Source: CAD feature listing. Evaluate the final solid. Frame: model axes, mm. A direction names the side the tool comes from. Coordinates: 2 decimals unless noted, no trailing zeros. Loops run counter-clockwise (first coordinate to the right, second up) from the corner with the lowest first, then second, coordinate; pieces in that order, holes last. Notation, with made-up numbers: M 6.25,27.5 L 60.25,27.5 A5 cw 60.25,32.5 Z; hole C -2.5,18.25 d11. An arc over 180 degrees is marked long. One line per question, with ' | ' between items. Start each with the question number.
1. Access query for faces 4 (the cylindrical face through (158.805, 91.82, 1.463)), 5 (the cylindrical face through (86.417, 17.759, 0.986)). Directions: +Z, -Z, +X, -X, +Y, -Y. A direction counts if a zero-diameter tool reaches every point of the face in a straight line with its end or side. Return the directions, or none.
2. Mould query, pull axis X, two halves, no side actions, for faces 1 (the cylindrical face through (168, 1, 1)), 2 (the flat face through (146.305, 76.981, 1.493)), 3 (the cylindrical face through (1, 2, 1)). Classes: pulls with the +X half, pulls with the -X half, needs draft (parallel to the pull), parting line crosses it, or undercut.
3. Section query A-A, the plane y = 17. Output: boundary loops of the cut face in (x, z), and give its area (3 significant figures).
4. Ray query, probe 1 along Y at (x, z) = (50, 1); probe 2 along X at (y, z) = (57.5, 1.6); probe 3 along X at (y, z) = (82.5, 0.9). Return the intervals inside material, ascending.
5. Section query C-C, the plane x = 50. Output: boundary loops of the cut face in (y, z).
6. Section query B-B, the plane x = 142.5. Output: boundary loops of the cut face in (y, z).
7. Section query D-D, the plane y = 83. Output: boundary loops of the cut face in (x, z), and give its area (3 significant figures).
Autodesk Fusion 360 part; units mm, degrees
sketch "Sketch1" plane through (0, 0, 0) normal (0, 0, 1) x (1, 0, 0)
  line L0 (0, 0) -> (170, 0)
  line L1 (170, 0) -> (170, 100)
  line L2 (170, 100) -> (0, 100)
  line L3 (0, 100) -> (0, 0)
  dimension "d1" = 170
  dimension "d2" = 100
extrude "Extrude1" add sketch "Sketch1" along normal blind 2 makes body 1
sketch "Sketch2" plane through (0, 0, 2) normal (0, 0, 1) x (-1, 0, 0)
  line L0 (0, -100) -> (0, 0)
  line L1 (0, 0) -> (-170, 0)
  line L2 (-170, 0) -> (-170, -100)
  line L3 (-170, -100) -> (0, -100)
  circle A0 centre (-17, -83) radius 3.5
  circle A1 centre (-50, -83) radius 3.5
  circle A2 centre (-83, -83) radius 3.5
  circle A3 centre (-17, -50) radius 3.5
  circle A4 centre (-50, -50) radius 3.5
  circle A5 centre (-83, -50) radius 3.5
  circle A6 centre (-17, -17) radius 3.5
  circle A7 centre (-50, -17) radius 3.5
  circle A8 centre (-83, -17) radius 3.5
  line L4 (-146.2, -23.8) -> (-160, -23.8)
  line L5 (-160, -23.8) -> (-160, -10)
  line L6 (-160, -10) -> (-146.2, -10)
  line L7 (-146.2, -10) -> (-146.2, -23.8)
  dimension "d5" = 7
  dimension "d9" = -66
  dimension "d10" = 66
  dimension "d11" = 100
  dimension "d12" = 33
  dimension "d13" = 17
  dimension "d14" = 17
  dimension "d15" = 17
  dimension "d16" = 13.8
  dimension "d17" = 13.8
  dimension "d18" = 10
  dimension "d19" = 10
sketch "Sketch3" plane through (0, 0, 2) normal (0, 0, 1) x (-1, 0, 0)
hole "Hole1" at (17, 83, 2) at (50, 83, 2) at (83, 83, 2) at (83, 50, 2) at (83, 17, 2) at (50, 17, 2) at (17, 17, 2) at (17, 50, 2) at (50, 50, 2) direction (0, 0, -1) diameter 7 depth 2 tip angle 180 bodies 1
sketch "Sketch4" plane through (0, 0, 2) normal (0, 0, 1) x (-1, 0, 0)
  line L0 (0, -100) -> (0, 0)
  line L1 (0, 0) -> (-170, 0)
  line L2 (-170, 0) -> (-170, -100)
  line L3 (-170, -100) -> (0, -100)
  circle A0 centre (-50, -50) radius 3.5
  circle A1 centre (-17, -17) radius 3.5
  circle A2 centre (-83, -17) radius 3.5
  circle A3 centre (-83, -83) radius 3.5
  circle A4 centre (-17, -83) radius 3.5
  circle A5 centre (-50, -83) radius 3.5
  circle A6 centre (-83, -50) radius 3.5
  circle A7 centre (-50, -17) radius 3.5
  circle A8 centre (-17, -50) radius 3.5
  line L4 (-160, -10) -> (-146.2, -10)
  line L5 (-146.2, -10) -> (-146.2, -23.8)
  line L6 (-146.2, -23.8) -> (-160, -23.8)
  line L7 (-160, -23.8) -> (-160, -10)
  dimension "d23" = 13.8
  dimension "d24" = 13.8
  dimension "d25" = 10
  dimension "d26" = 10
sketch "Sketch5" plane through (0, 0, 2) normal (0, 0, 1) x (-1, 0, 0)
extrude "Extrude2" cut sketch "Sketch4" against normal blind 2 contours L4 L5 L6 L7 bodies 1
pattern_linear "R-Pattern1" count 3 spacing 21 along (-1, 0, 0) count 3 spacing 21 along (0, 1, 0) of "Extrude2"
sketch "Sketch6" plane through (0, 0, 2) normal (0, 0, 1) x (-1, 0, 0)
  line L0 (-146.2, -10) -> (-146.2, -23.8)
  line L1 (-146.2, -23.8) -> (-160, -23.8)
  line L2 (-160, -23.8) -> (-160, -10)
  line L3 (-160, -10) -> (-146.2, -10)
  line L4 (0, -100) -> (0, 0)
  line L5 (0, 0) -> (-170, 0)
  line L6 (-170, 0) -> (-170, -100)
  line L7 (-170, -100) -> (0, -100)
  circle A0 centre (-50, -50) radius 3.5
  circle A1 centre (-17, -17) radius 3.5
  circle A2 centre (-83, -17) radius 3.5
  circle A3 centre (-83, -83) radius 3.5
  circle A4 centre (-17, -83) radius 3.5
  circle A5 centre (-50, -83) radius 3.5
  circle A6 centre (-83, -50) radius 3.5
  circle A7 centre (-50, -17) radius 3.5
  circle A8 centre (-17, -50) radius 3.5
  line L8 (-125.2, -10) -> (-125.2, -23.8)
  line L9 (-125.2, -23.8) -> (-139, -23.8)
  line L10 (-139, -23.8) -> (-139, -10)
  line L11 (-139, -10) -> (-125.2, -10)
  line L12 (-104.2, -10) -> (-104.2, -23.8)
  line L13 (-104.2, -23.8) -> (-118, -23.8)
  line L14 (-118, -23.8) -> (-118, -10)
  line L15 (-118, -10) -> (-104.2, -10)
  line L16 (-146.2, -31) -> (-146.2, -44.8)
  line L17 (-146.2, -44.8) -> (-160, -44.8)
  line L18 (-160, -44.8) -> (-160, -31)
  line L19 (-160, -31) -> (-146.2, -31)
  line L20 (-125.2, -31) -> (-125.2, -44.8)
  line L21 (-125.2, -44.8) -> (-139, -44.8)
  line L22 (-139, -44.8) -> (-139, -31)
  line L23 (-139, -31) -> (-125.2, -31)
  line L24 (-104.2, -31) -> (-104.2, -44.8)
  line L25 (-104.2, -44.8) -> (-118, -44.8)
  line L26 (-118, -44.8) -> (-118, -31)
  line L27 (-118, -31) -> (-104.2, -31)
  line L28 (-146.2, -52) -> (-146.2, -65.8)
  line L29 (-146.2, -65.8) -> (-160, -65.8)
  line L30 (-160, -65.8) -> (-160, -52)
  line L31 (-160, -52) -> (-146.2, -52)
  line L32 (-125.2, -52) -> (-125.2, -65.8)
  line L33 (-125.2, -65.8) -> (-139, -65.8)
  line L34 (-139, -65.8) -> (-139, -52)
  line L35 (-139, -52) -> (-125.2, -52)
  line L36 (-104.2, -52) -> (-104.2, -65.8)
  line L37 (-104.2, -65.8) -> (-118, -65.8)
  line L38 (-118, -65.8) -> (-118, -52)
  line L39 (-118, -52) -> (-104.2, -52)
  circle A9 centre (-83, -17) radius 10.5
  dimension "d33" = 21
sketch "Sketch7" plane through (0, 0, 2) normal (0, 0, 1) x (-1, 0, 0)
  line L0 (-133, -96.2) -> (-160, -96.2)
  line L1 (-160, -96.2) -> (-160, -69.2)
  line L2 (-160, -69.2) -> (-133, -69.2)
  line L3 (-133, -69.2) -> (-133, -96.2)
  line L4 (-170, -100) -> (0, -100)
  line L5 (-160, -10) -> (-146.2, -10)
  line L6 (0, 0) -> (-170, 0)
  line L7 (-136, -90) -> (-157, -90)
  line L8 (-157, -90) -> (-157, -79.2)
  line L9 (-157, -79.2) -> (-136, -79.2)
  line L10 (-136, -79.2) -> (-136, -90)
  line L11 (-170, 0) -> (-170, -100)
  line L12 (-146.2, -65.8) -> (-160, -65.8)
  dimension "d36" = 27
  dimension "d37" = 27
  dimension "d38" = 3.8
  dimension "d39" = 10
  dimension "d40" = 3
  dimension "d42" = 10.8
  dimension "d43" = 21
  dimension "d53" = 10
  dimension "d55" = 10
  dimension "d67" = 6.2
  dimension "d68" = 10
  dimension "d69" = 3.4
extrude "Extrude3" cut sketch "Sketch7" against normal blind 2 contours L7 L8 L9 L10 bodies 1
chamfer "Chamfer1" distance 4.5 distance2 1 4 edges at (146.5, 90, 2) (136, 84.6, 2) (146.5, 79.2, 2) (157, 84.6, 2) measured on face at (108.8707, 79.8596, 2) measured on face at (108.8707, 79.8596, 2) measured on face at (108.8707, 79.8596, 2) measured on face at (108.8707, 79.8596, 2) on bodies 1
sketch "Sketch8" plane through (0, 0, 2) normal (0, 0, 1) x (-1, 0, 0)
  line L0 (-104.2, -86.8) -> (-118, -86.8)
  line L1 (-118, -86.8) -> (-118, -73)
  line L2 (-118, -73) -> (-104.2, -73)
  line L3 (-104.2, -73) -> (-104.2, -86.8)
  line L4 (-118, -52) -> (-104.2, -52)
  line L5 (-125.2, -52) -> (-125.2, -65.8)
  point P0 (-104.2, -10)
  point P1 (-125.2, -10)
  dimension "d48" = 21
  dimension "d49" = 21
  dimension "d50" = 21
  dimension "d51" = 13.8
  dimension "d52" = 13.8
extrude "Extrude4" cut sketch "Sketch8" against normal blind 2 bodies 1
sketch "Sketch9" plane through (0, 0, 2) normal (0, 0, 1) x (-1, 0, 0)
  line L0 (-125.2, -65.8) -> (-139, -65.8)
  line L1 (-118, -73) -> (-104.2, -73)
  line L2 (-104.2, -65.8) -> (-118, -65.8)
  dimension "d61" = 7.2
fillet "Fillet1" radius 5 4 edges at (170, 0, 1) (170, 100, 1) (0, 0, 1) (0, 100, 1) on bodies 1
fillet "Fillet2" radius 5 4 edges at (133.75, 92.25, 1.5) (133.75, 76.95, 1.5) (159.25, 92.25, 1.5) (159.25, 76.95, 1.5) on bodies 1
sketch "Sketch10" plane through (0, 0, 2) normal (0, 0, 1) x (-1, 0, 0)
  line L0 (-5, 0) -> (-165, 0)
  line L1 (-170, -5) -> (-170, -95)
  line L2 (-165, -100) -> (-5, -100)
  line L3 (0, -95) -> (0, -5)
  line L4 (-3, -102) -> (-167, -102)
  line L5 (-172, -97) -> (-172, -3)
  line L6 (-167, 2) -> (-3, 2)
  line L7 (2, -3) -> (2, -97)
  arc A0 (-5, -100) -> (0, -95) centre (-5, -95) ccw
  arc A1 (-170, -95) -> (-165, -100) centre (-165, -95) ccw
  arc A2 (-165, 0) -> (-170, -5) centre (-165, -5) ccw
  arc A3 (0, -5) -> (-5, 0) centre (-5, -5) ccw
  arc A4 (2, -3) -> (-3, 2) centre (-3, -3) ccw
  arc A5 (-3, -102) -> (2, -97) centre (-3, -97) ccw
  arc A6 (-172, -97) -> (-167, -102) centre (-167, -97) ccw
  arc A7 (-167, 2) -> (-172, -3) centre (-167, -3) ccw
  dimension "d70" = 2
  dimension "d71" = 2
  dimension "d72" = 2
  dimension "d73" = 2
  dimension "d74" = 5
extrude "Extrude5" add sketch "Sketch10" along normal blind 50 separate body makes body 2
move_face "OffsetFaces1" offset 2 1 faces at (58.3333, -1.3333, 2) on bodies 2
sketch "Sketch11" plane through (0, 100, 0) normal (0, -1, 0) x (1, 0, 0)
  line L0 (5, 0) -> (165, 0)
  line L1 (165, 0) -> (165, 52)
  line L2 (165, 52) -> (5, 52)
  line L3 (5, 52) -> (5, 0)
  line L4 (165, 0.1269) -> (161.7551, 0.1269)
  line L5 (161.7551, 0.1269) -> (161.7551, 2.1269)
  line L6 (161.7551, 2.1269) -> (165, 2.1269)
  line L7 (165, 2.1269) -> (165, 0.1269)
  line L8 (161.7551, 2.1269) -> (156.7551, 2.1269)
  line L9 (156.7551, 2.1269) -> (156.7551, 4.1269)
  line L10 (156.7551, 4.1269) -> (161.7551, 4.1269)
  line L11 (161.7551, 4.1269) -> (161.7551, 2.1269)
  dimension "d78" = 2
  dimension "d79" = 5
  dimension "d80" = 2
  dimension "d81" = 160
hidden bodies 2
Taken from the geometry:
1) face 4: +Z | face 5: +Z, -Z
2) face 1: pulls with the +X half | face 2: undercut | face 3: pulls with the -X half
3) outline: M 0,0 L 13.5,0 L 13.5,2 L 0,2 Z; M 20.5,0 L 46.5,0 L 46.5,2 L 20.5,2 Z; M 53.5,0 L 79.5,0 L 79.5,2 L 53.5,2 Z; M 86.5,0 L 104.2,0 L 104.2,2 L 86.5,2 Z; M 118,0 L 125.2,0 L 125.2,2 L 118,2 Z; M 139,0 L 146.2,0 L 146.2,2 L 139,2 Z; M 160,0 L 170,0 L 170,2 L 160,2 Z | area: 215 mm^2
4) probe 1: 0 to 13.5, 20.5 to 46.5, 53.5 to 79.5, 86.5 to 100 | probe 2: 0 to 104.2, 118 to 125.2, 139 to 146.2, 160 to 170 | probe 3: 0 to 13.54, 20.46 to 46.54, 53.46 to 79.54, 86.46 to 104.2, 118 to 136, 157 to 170
5) outline: M 0,0 L 13.5,0 L 13.5,2 L 0,2 Z; M 20.5,0 L 46.5,0 L 46.5,2 L 20.5,2 Z; M 53.5,0 L 79.5,0 L 79.5,2 L 53.5,2 Z; M 86.5,0 L 100,0 L 100,2 L 86.5,2 Z
6) outline: M 0,0 L 79.2,0 L 79.2,1 L 74.7,2 L 0,2 Z; M 90,0 L 100,0 L 100,2 L 94.5,2 L 90,1 Z
7) outline: M 0,0 L 13.5,0 L 13.5,2 L 0,2 Z; M 20.5,0 L 46.5,0 L 46.5,2 L 20.5,2 Z; M 53.5,0 L 79.5,0 L 79.5,2 L 53.5,2 Z; M 86.5,0 L 104.2,0 L 104.2,2 L 86.5,2 Z; M 118,0 L 136,0 L 136,1 L 131.5,2 L 118,2 Z; M 157,0 L 170,0 L 170,2 L 161.5,2 L 157,1 Z | area: 224 mm^2
